```python
from build123d import *

# Parameters (mm, degrees)
F1_DEPTH = 150
F3_D     = 3
F4_D     = 8


with BuildPart() as f1:
    # F0 (on Right) → F1 (new body)
    with BuildSketch(Plane.YZ):
        Polygon((0, 23.237994), (0, 43.237994), (-19, 43.237994), (-19, -36.762006), (0, -36.762006), (0, -16.762006), (-6, -16.762006), (-6, 23.237994), align=None)
    extrude(amount=F1_DEPTH)

    # F3 (through all)
    with Locations(Plane.XZ.offset(19)):
        with Locations((12, 29.237994), (138, 29.237994), (12, -22.762006), (138, -22.762006), (118, 29.237994), (118, -22.762006), (32, 29.237994), (32, -22.762006)):
            Hole(F3_D / 2)

    # F4 (through all)
    with Locations(Plane.XZ.offset(19)):
        with Locations((128, 36.237994), (22, 36.237994), (22, -29.762006), (128, -29.762006)):
            Hole(F4_D / 2)


solid = f1.part
```
Work out the finished part from the listing and answer in its coordinate system (mm). A direction names the side the tool comes from. Coordinates: 2 decimals unless noted, no trailing zeros. Order: outer loops, then holes, each group sorted by start corner. A loop starts at its lowest first (then second) coordinate and runs counter-clockwise, first axis right, second up. Notation, with made-up numbers: M 52,-30.75 L 69,-30.75 A24 cw 69,7.25 Z; hole C -26,51 d3. An arc over 180 degrees is marked long. Use CSV: the item, a comma, the result in double quotes.
1) Section B-B on y = -15.75 is taken. Count the separate pieces of the cut face and the enclosed holes in it, plus the area to 3 significant figures.
Worked out:
separate pieces,"1"
enclosed holes,"12"
area,"11,700 mm^2"
2) For faces 4 (the face through (12.325, -9.367, 27.774)), 5 (the face through (74, -6, 3)), determine the directions among +Z, -Z, +X, -X, +Y, -Y from which every point of the face is accessible in a straight line to the end or side of a thin tool.
Worked out:
face 4,"+Y, -Y"
face 5,"+X, -X, +Y"
3) Consider line 1 (X direction, y = -9.75, z = 36.5); line 2 (Z direction, x = 118, y = -7.5); line 3 (Z direction, x = 29, y = -3.25). Determine where each line is inside the solid, lowest interval first. Write a range as [from, to].
Worked out:
line 1,"x = [0, 18.01], [25.99, 124.01], [131.99, 150]"
line 2,"z = [-36.76, -24.26], [-21.26, 27.74], [30.74, 43.24]"
line 3,"z = [-36.76, -16.76], [23.24, 43.24]"
4) Determine the mould class of faces 1 (the face through (12.325, -9.367, -24.226)), 2 (the face through (74, 0, 33)), 3 (the face through (74, -10, -36.762)) for opening direction Z: released by +Z, released by -Z, zero draft, split by the parting line, or undercut.
Worked out:
face 1,"undercut"
face 2,"zero draft"
face 3,"released by -Z"
5) Section D-D on x = 39.5 is taken. Write down the section's boundary in (y, z), plus the area to 3 significant figures.
Worked out:
outline,"M -19,-36.76 L 0,-36.76 L 0,-16.76 L -6,-16.76 L -6,23.24 L 0,23.24 L 0,43.24 L -19,43.24 Z"
area,"1,280 mm^2"
6) Section A-A on x = 128 is taken. Write down the section's boundary in (y, z).
Worked out:
outline,"M -19,-36.76 L 0,-36.76 L 0,-33.76 L -19,-33.76 Z; M -19,-25.76 L 0,-25.76 L 0,-16.76 L -6,-16.76 L -6,23.24 L 0,23.24 L 0,32.24 L -19,32.24 Z; M -19,40.24 L 0,40.24 L 0,43.24 L -19,43.24 Z"
